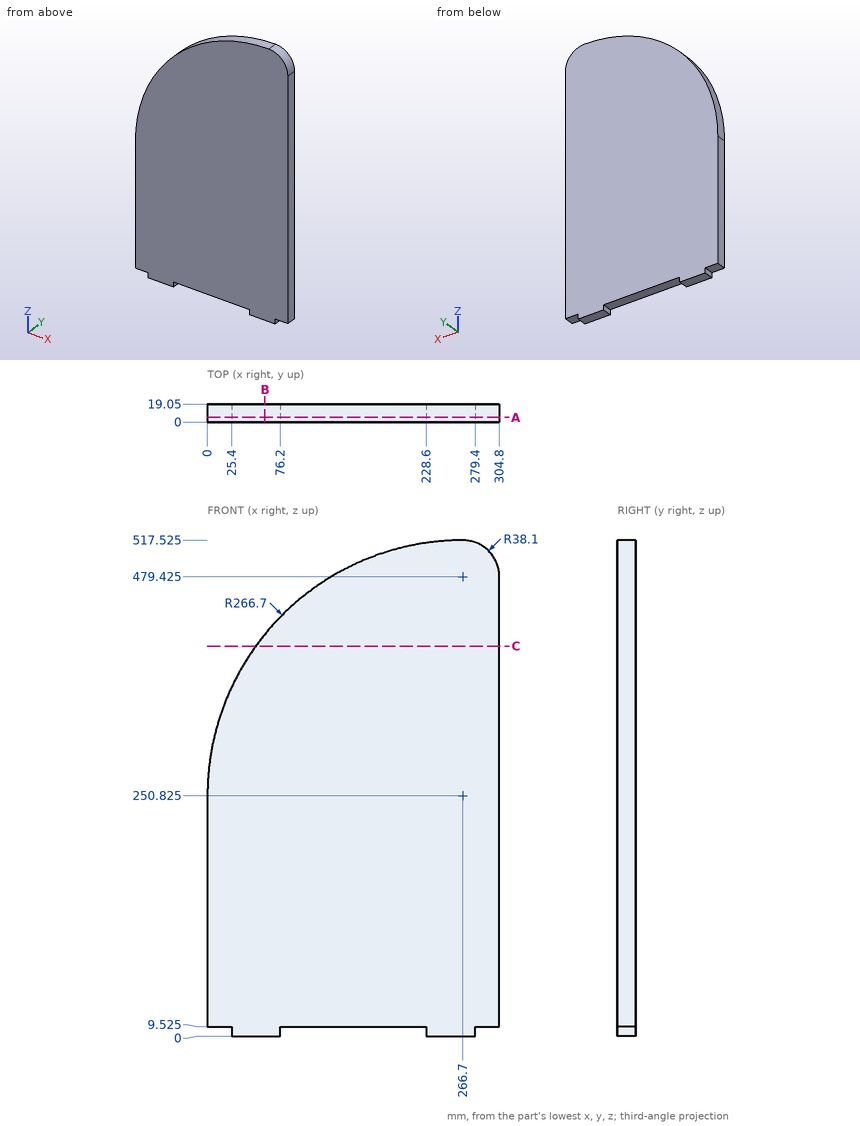
Design review of the part shown in the three views and the two pictorial views. Dimensions are in mm from the part's minimum x, y and z. Coordinates: 2 decimals unless noted, no trailing zeros. Loops run counter-clockwise (first coordinate to the right, second up) from the corner with the lowest first, then second, coordinate; pieces in that order, holes last.
Q1. We need section B-B on x = 60. State the section outline as (y, z) points, and give its area (3 significant figures).
Reported:
outline: (0, 0) - (19.05, 0) - (19.05, 419.36) - (0, 419.36) - close
area: 7,990 mm2
Q2. For pin 1 (7.5 mm diameter, centred on y = 5, z = 3.5, fed in from +X); pin 2 (1 mm diameter, centred on x = 80, y = 16.5, fed in from -Z) (3 decimals); pin 3 (7.5 mm diameter, centred on y = 6.5, z = 3.5, fed in from -X), all flat-tipped, find the tip position at first contact; note any pin that passes through.
Reported:
pin 1: stops at x = 279.4
pin 2: stops at z = 9.525
pin 3: stops at x = 25.4
Q3. We need section A-A on y = 5. State the section outline as (x, z) points (3 decimals), and give its area (3 significant figures).
Reported:
outline: (0, 9.525) - (25.4, 9.525) - (25.4, 0) - (76.2, 0) - (76.2, 9.525) - (228.6, 9.525) - (228.6, 0) - (279.4, 0) - (279.4, 9.525) - (304.8, 9.525) - (304.8, 479.425) arc R38.1 ccw to (266.7, 517.525) arc R266.7 ccw to (0, 250.825) - close
area: 140,000 mm2
Q4. To check wall thickness, follow line 1 (X direction, y = 17.25, z = 456.5); line 2 (Z direction, x = 191, y = 12.5) (3 decimals); line 3 (X direction, y = 11, z = 319). State the ranges of each line that lie inside material, in increasing order.
Reported:
line 1: x = 96.92 to 304.8
line 2: z = 9.525 to 506.556
line 3: x = 8.86 to 304.8
Q5. We need section C-C on z = 407. State the section outline as (x, y) points.
Reported:
outline: (50.51, 0) - (304.8, 0) - (304.8, 19.05) - (50.51, 19.05) - close
